Build history of the part. All positions in model axes, mm. Face numbers are marked on the shaded views. Round coordinates to 2 decimals unless told otherwise and drop trailing zeros. Write each loop counter-clockwise with the first axis right and the second up, starting at its lowest first coordinate (ties: lowest second). Pieces come first, ordered by that corner, then holes. Notation, with made-up numbers: M -30,10.25 L 17,10.25 A16 ccw 17,26.25 Z; hole C 20.25,30.5 d2. An arc over 180 degrees is marked long. Use a Markdown table: item, result.
from build123d import *

# Parameters (mm, degrees)
SKETCH085_R     = 100
SKETCH085_R_2   = 1.6
PAD029_DEPTH    = 10
SKETCH086_R     = 32.5
POCKET051_DEPTH = 8
SKETCH087_R     = 4.5
POCKET052_DEPTH = 5
CHAMFER009_SIZE = 1


with BuildPart() as part:
    # Sketch085 → Pad029 (new body)
    with BuildSketch(Plane.XY):
        Circle(SKETCH085_R)
        with Locations((-18, 90.4921108583)):
            Circle(SKETCH085_R_2, mode=Mode.SUBTRACT)
        with Locations((18, 90.4921108583)):
            Circle(SKETCH085_R_2, mode=Mode.SUBTRACT)
        with Locations((51.2596631704, 76.7155072931)):
            Circle(SKETCH085_R_2, mode=Mode.SUBTRACT)
        with Locations((76.7155072931, 51.2596631704)):
            Circle(SKETCH085_R_2, mode=Mode.SUBTRACT)
        with Locations((90.4921108583, 18)):
            Circle(SKETCH085_R_2, mode=Mode.SUBTRACT)
        with Locations((90.4921108583, -18)):
            Circle(SKETCH085_R_2, mode=Mode.SUBTRACT)
        with Locations((76.7155072931, -51.2596631704)):
            Circle(SKETCH085_R_2, mode=Mode.SUBTRACT)
        with Locations((51.2596631704, -76.7155072931)):
            Circle(SKETCH085_R_2, mode=Mode.SUBTRACT)
        with Locations((18, -90.4921108583)):
            Circle(SKETCH085_R_2, mode=Mode.SUBTRACT)
        with Locations((-18, -90.4921108583)):
            Circle(SKETCH085_R_2, mode=Mode.SUBTRACT)
        with Locations((-51.2596631704, -76.7155072931)):
            Circle(SKETCH085_R_2, mode=Mode.SUBTRACT)
        with Locations((-76.7155072931, -51.2596631704)):
            Circle(SKETCH085_R_2, mode=Mode.SUBTRACT)
        with Locations((-90.4921108583, -18)):
            Circle(SKETCH085_R_2, mode=Mode.SUBTRACT)
        with Locations((-90.4921108583, 18)):
            Circle(SKETCH085_R_2, mode=Mode.SUBTRACT)
        with Locations((-76.7155072931, 51.2596631704)):
            Circle(SKETCH085_R_2, mode=Mode.SUBTRACT)
        with Locations((-51.2596631704, 76.7155072931)):
            Circle(SKETCH085_R_2, mode=Mode.SUBTRACT)
        with Locations((-75.4100923819, 15)):
            Circle(SKETCH085_R_2, mode=Mode.SUBTRACT)
        with Locations((-75.4100923819, -15)):
            Circle(SKETCH085_R_2, mode=Mode.SUBTRACT)
        with Locations((-63.9295894109, -42.7163859753)):
            Circle(SKETCH085_R_2, mode=Mode.SUBTRACT)
        with Locations((-42.7163859753, -63.9295894109)):
            Circle(SKETCH085_R_2, mode=Mode.SUBTRACT)
        with Locations((-15, -75.4100923819)):
            Circle(SKETCH085_R_2, mode=Mode.SUBTRACT)
        with Locations((15, -75.4100923819)):
            Circle(SKETCH085_R_2, mode=Mode.SUBTRACT)
        with Locations((42.7163859753, -63.9295894109)):
            Circle(SKETCH085_R_2, mode=Mode.SUBTRACT)
        with Locations((63.9295894109, -42.7163859753)):
            Circle(SKETCH085_R_2, mode=Mode.SUBTRACT)
        with Locations((75.4100923819, -15)):
            Circle(SKETCH085_R_2, mode=Mode.SUBTRACT)
        with Locations((75.4100923819, 15)):
            Circle(SKETCH085_R_2, mode=Mode.SUBTRACT)
        with Locations((63.9295894109, 42.7163859753)):
            Circle(SKETCH085_R_2, mode=Mode.SUBTRACT)
        with Locations((42.7163859753, 63.9295894109)):
            Circle(SKETCH085_R_2, mode=Mode.SUBTRACT)
        with Locations((15, 75.4100923819)):
            Circle(SKETCH085_R_2, mode=Mode.SUBTRACT)
        with Locations((-15, 75.4100923819)):
            Circle(SKETCH085_R_2, mode=Mode.SUBTRACT)
        with Locations((-42.7163859753, 63.9295894109)):
            Circle(SKETCH085_R_2, mode=Mode.SUBTRACT)
        with Locations((-63.9295894109, 42.7163859753)):
            Circle(SKETCH085_R_2, mode=Mode.SUBTRACT)
        with Locations((-34.1731089215, 51.1436717401)):
            Circle(SKETCH085_R_2, mode=Mode.SUBTRACT)
        with Locations((-12.0000000496, 60.3280741548)):
            Circle(SKETCH085_R_2, mode=Mode.SUBTRACT)
        with Locations((12.0000000496, 60.3280741548)):
            Circle(SKETCH085_R_2, mode=Mode.SUBTRACT)
        with Locations((34.1731089215, 51.1436717401)):
            Circle(SKETCH085_R_2, mode=Mode.SUBTRACT)
        with Locations((51.1436717401, 34.1731089215)):
            Circle(SKETCH085_R_2, mode=Mode.SUBTRACT)
        with Locations((60.3280741548, 12.0000000496)):
            Circle(SKETCH085_R_2, mode=Mode.SUBTRACT)
        with Locations((60.3280741548, -12.0000000496)):
            Circle(SKETCH085_R_2, mode=Mode.SUBTRACT)
        with Locations((51.1436717401, -34.1731089215)):
            Circle(SKETCH085_R_2, mode=Mode.SUBTRACT)
        with Locations((34.1731089215, -51.1436717401)):
            Circle(SKETCH085_R_2, mode=Mode.SUBTRACT)
        with Locations((12.0000000496, -60.3280741548)):
            Circle(SKETCH085_R_2, mode=Mode.SUBTRACT)
        with Locations((-12.0000000496, -60.3280741548)):
            Circle(SKETCH085_R_2, mode=Mode.SUBTRACT)
        with Locations((-34.1731089215, -51.1436717401)):
            Circle(SKETCH085_R_2, mode=Mode.SUBTRACT)
        with Locations((-51.1436717401, -34.1731089215)):
            Circle(SKETCH085_R_2, mode=Mode.SUBTRACT)
        with Locations((-60.3280741548, -12.0000000496)):
            Circle(SKETCH085_R_2, mode=Mode.SUBTRACT)
        with Locations((-60.3280741548, 12.0000000496)):
            Circle(SKETCH085_R_2, mode=Mode.SUBTRACT)
        with Locations((-51.1436717401, 34.1731089215)):
            Circle(SKETCH085_R_2, mode=Mode.SUBTRACT)
        with Locations((-25.6298315852, 38.3577536466)):
            Circle(SKETCH085_R_2, mode=Mode.SUBTRACT)
        with Locations((-9, 45.2460554291)):
            Circle(SKETCH085_R_2, mode=Mode.SUBTRACT)
        with Locations((9, 45.2460554291)):
            Circle(SKETCH085_R_2, mode=Mode.SUBTRACT)
        with Locations((25.6298315852, 38.3577536466)):
            Circle(SKETCH085_R_2, mode=Mode.SUBTRACT)
        with Locations((38.3577536466, 25.6298315852)):
            Circle(SKETCH085_R_2, mode=Mode.SUBTRACT)
        with Locations((45.2460554291, 9)):
            Circle(SKETCH085_R_2, mode=Mode.SUBTRACT)
        with Locations((45.2460554291, -9)):
            Circle(SKETCH085_R_2, mode=Mode.SUBTRACT)
        with Locations((38.3577536466, -25.6298315852)):
            Circle(SKETCH085_R_2, mode=Mode.SUBTRACT)
        with Locations((25.6298315852, -38.3577536466)):
            Circle(SKETCH085_R_2, mode=Mode.SUBTRACT)
        with Locations((9, -45.2460554291)):
            Circle(SKETCH085_R_2, mode=Mode.SUBTRACT)
        with Locations((-9, -45.2460554291)):
            Circle(SKETCH085_R_2, mode=Mode.SUBTRACT)
        with Locations((-25.6298315852, -38.3577536466)):
            Circle(SKETCH085_R_2, mode=Mode.SUBTRACT)
        with Locations((-38.3577536466, -25.6298315852)):
            Circle(SKETCH085_R_2, mode=Mode.SUBTRACT)
        with Locations((-45.2460554291, -9)):
            Circle(SKETCH085_R_2, mode=Mode.SUBTRACT)
        with Locations((-45.2460554291, 9)):
            Circle(SKETCH085_R_2, mode=Mode.SUBTRACT)
        with Locations((-38.3577536466, 25.6298315852)):
            Circle(SKETCH085_R_2, mode=Mode.SUBTRACT)
    extrude(amount=PAD029_DEPTH)

    # Sketch086 (on Face66 of Pad029) → Pocket051 (cut)
    with BuildSketch(Plane(origin=(0, 0, 0), x_dir=(1, 0, 0), z_dir=(0, 0, -1))):
        Circle(SKETCH086_R)
    extrude(amount=-POCKET051_DEPTH, mode=Mode.SUBTRACT)

    # Sketch087 (on Face3 of Pocket051) → Pocket052 (cut)
    with BuildSketch(Plane.XY.offset(10)):
        Circle(SKETCH087_R)
    extrude(amount=-POCKET052_DEPTH, mode=Mode.SUBTRACT)

    # Chamfer009
    chamfer009_edges = [part.edges().sort_by_distance(p)[0] for p in [
        (-32.5, 0, 0),
    ]]
    chamfer(chamfer009_edges, length=CHAMFER009_SIZE)


solid = part.part
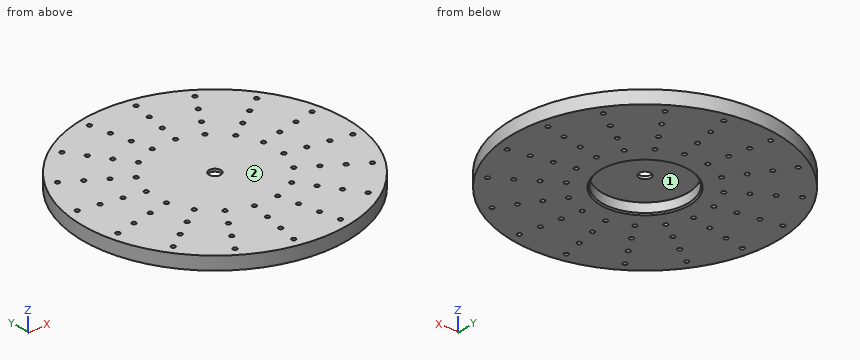
Q1. Cut at B-B on x = -85. Give the cut face in (y, z).
Response values:
| item | result |
|---|---|
| outline | M -52.68,0 L 52.68,0 L 52.68,10 L -52.68,10 Z |
Q2. Two-plate mould, pull along Y, no slides. Class the marked faces 1 and 2: +Y half, -Y half, draft (parallel to the pull), parting line (faces both ways), or undercut.
Response values:
| item | result |
|---|---|
| face 1 | undercut |
| face 2 | draft |
Q3. Drop flat-ended pins along their axis: P1, Ø5, axis at y = 14.5, z = 1, coming from the +X side; P2, Ø3, axis at x = 18.5, y = -24, coming from the -Z side; P3, Ø4, axis at y = -71.5, z = 4, coming from the -X side. Give the stop position or say it passes through.
Response values:
| item | result |
|---|---|
| P1 | stops at x = 99.28 |
| P2 | stops at z = 8 |
| P3 | stops at x = -71.9 |
Q4. Drill centre lines: L1, parallel to X at y = 35, z = 3.75; L2, parallel to Y at x = 60, z = 4.75; L3, parallel to X at y = 14, z = 6.75. Where is each one in solid material? Low to high.
Response values:
| item | result |
|---|---|
| L1 | x = -93.67 to -52.51, -49.77 to 49.77, 52.51 to 93.67 |
| L2 | y = -80 to -13.57, -10.43 to 10.43, 13.57 to 80 |
| L3 | x = -99.02 to -76.66, -74.16 to -29.33, 29.33 to 74.16, 76.66 to 99.02 |
Q5. Cut at A-A on z = 4. Count the separate pieces of the cut face and the enclosed holes in it, and give its area (3 significant figures).
Response values:
| item | result |
|---|---|
| separate pieces | 1 |
| enclosed holes | 65 |
| area | 27,600 mm2 |
